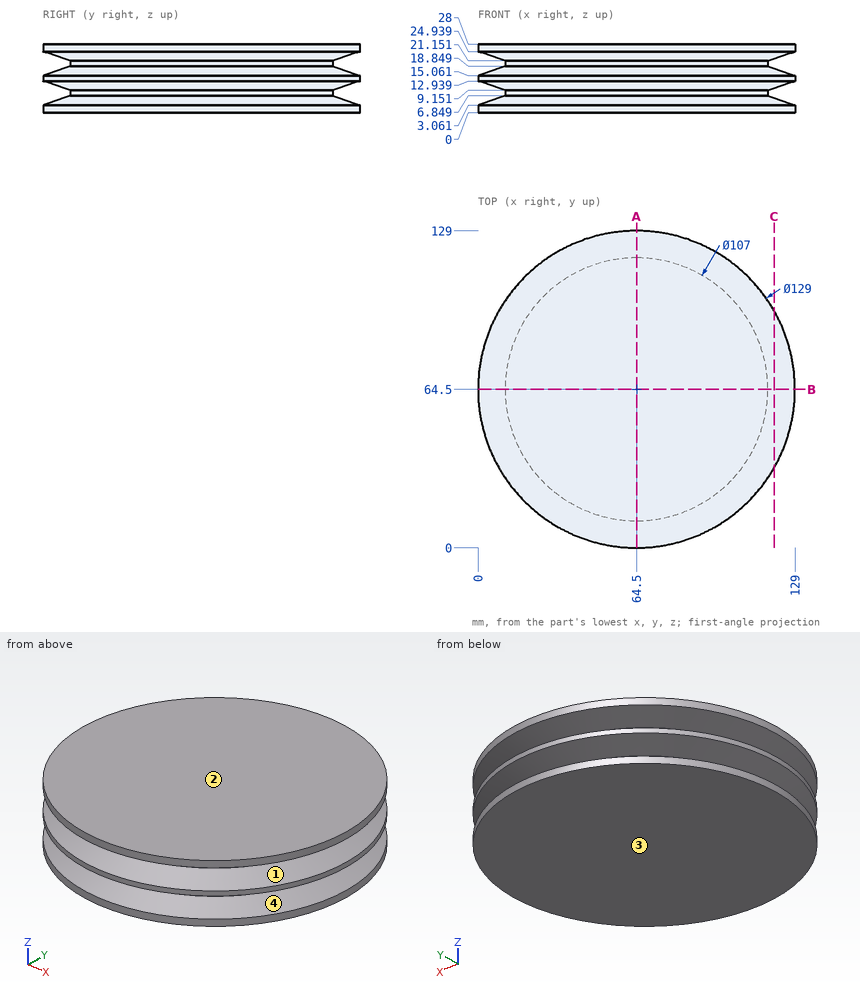
Drawing for the job (mm, zero at the part's lowest x, y, z). Give positions to 0.01 mm unless a question says otherwise; leave off trailing zeros. Loops run counter-clockwise (first coordinate to the right, second up) from the corner with the lowest first, then second, coordinate; pieces in that order, holes last.
(1) Drill centre lines: line 1 along Z through (x, y) = (75.5, 8); line 2 along X through (y, z) = (63.5, 26); line 3 along X through (y, z) = (97.5, 19.5). Where is each one in solid material? Low to high.
Return value:
line 1: z = 0 to 5.45, 10.55 to 17.45, 22.55 to 28
line 2: x = 0.01 to 128.99
line 3: x = 22.39 to 106.61
(2) Pin check, flat tips, straight feed: pin 1 (1.5 mm diameter, centred on x = 33, y = 113, fed in from -Z); pin 2 (8 mm diameter, centred on x = 106, z = 16.5, fed in from +Y); pin 3 (4 mm diameter, centred on y = 53, z = 11.5, fed in from +X); pin 4 (6 mm diameter, centred on x = 45, z = 4, fed in from +Y). Stop position of each tip, or through.
Return value:
pin 1: stops at z = 0
pin 2: stops at y = 116.79
pin 3: stops at x = 128.2
pin 4: stops at y = 126.81
(3) Pull direction Z, two halves, no side cores. Call the marked faces 1, 2, 3 and 4: pulls with the +Z half, pulls with the -Z half, needs draft (parallel to the pull), parting line crosses it, or undercut.
Return value:
face 1: undercut
face 2: pulls with the +Z half
face 3: pulls with the -Z half
face 4: undercut
(4) Band-saw the part on C-C (x = 120.5). Count the separate pieces of the cut face and the enclosed holes in it, and give its area (3 significant figures).
Return value:
separate pieces: 3
enclosed holes: 0
area: 1,020 mm2
(5) Band-saw the part on A-A (x = 64.5). Write the cut outline in (y, z).
Return value:
outline: (0, 0) - (129, 0) - (129, 3.06) - (118, 6.85) - (118, 9.15) - (129, 12.94) - (129, 15.06) - (118, 18.85) - (118, 21.15) - (129, 24.94) - (129, 28) - (0, 28) - (0, 24.94) - (11, 21.15) - (11, 18.85) - (0, 15.06) - (0, 12.94) - (11, 9.15) - (11, 6.85) - (0, 3.06) - close
